Model file for the job. Use its own axes, mm. A direction names the side the tool comes from. Coordinates: 2 decimals unless noted, no trailing zeros. Loops run counter-clockwise (first coordinate to the right, second up) from the corner with the lowest first, then second, coordinate; pieces in that order, holes last.
from build123d import *
from build123d.topology import SkipClean

# Parameters (mm, degrees)
SKETCH1_R           = 6.35
BOSS_EXTRUDE1_DEPTH = 2.45
SKETCH2_R           = 1.5
BOSS_EXTRUDE2_DEPTH = 2.45
SKETCH3_R           = 2.85
CUT_EXTRUDE1_DEPTH  = 1.8
CHAMFER1_SIZE       = 5
CHAMFER1_SIZE2      = 3.501037691
BOSS_EXTRUDE3_DEPTH = 7.85


with BuildPart() as part:
    # Sketch1 → Boss-Extrude1 (new body)
    with BuildSketch(Plane(origin=(0, 0, 0), x_dir=(1, 0, 0), z_dir=(0, 1, 0))):
        with BuildLine():
            Line((-14.3, -17.6), (14.3, -17.6))
            Line((14.3, -17.6), (14.3, 5.715767665))
            ThreePointArc((14.3, 5.715767665), (0, 15.4), (-14.3, 5.715767665))
            Line((-14.3, 5.715767665), (-14.3, -17.6))
        make_face()
        with Locations(Location((0, 0, 0), (0, 0, 270))):
            Circle(SKETCH1_R, mode=Mode.SUBTRACT)
    extrude(amount=BOSS_EXTRUDE1_DEPTH)

    # Sketch2 → Boss-Extrude2 (add)
    with BuildSketch(Plane(origin=(0, 0, 0), x_dir=(1, 0, 0), z_dir=(0, 1, 0))):
        with BuildLine():
            ThreePointArc((24.104102849, -3.187555227), (26.549963246, 0.015574774), (24.073976981, 3.195475228))
            Line((24.073976981, 3.195475228), (14.3, 5.715767665))
            Line((14.3, 5.715767665), (14.3, -5.814556668))
            Line((14.3, -5.814556668), (24.104102849, -3.187555227))
        make_face()
        with Locations(Location((16.25, 0, 0), (0, 0, 270))):
            Circle(SKETCH2_R, mode=Mode.SUBTRACT)
        with Locations(Location((23.25, 0, 0), (0, 0, 270))):
            Circle(SKETCH2_R, mode=Mode.SUBTRACT)
    boss_extrude2 = extrude(amount=BOSS_EXTRUDE2_DEPTH)

    # Sketch3 → Cut-Extrude1 (cut)
    with BuildSketch(Plane(origin=(0, 2.45, 0), x_dir=(1, 0, 0), z_dir=(0, 1, 0))):
        with Locations(Location((16.25, 0, 0), (0, 0, 270))):
            Circle(SKETCH3_R)
    cut_extrude1 = extrude(amount=-CUT_EXTRUDE1_DEPTH, mode=Mode.SUBTRACT)

    # Mirror1: Boss-Extrude2, Cut-Extrude1 across plane
    add(boss_extrude2.mirror(Plane(origin=(0, 0, 0), x_dir=(0, 0, 1), z_dir=(1, 0, 0))))
    add(cut_extrude1.mirror(Plane(origin=(0, 0, 0), x_dir=(0, 0, 1), z_dir=(1, 0, 0))), mode=Mode.SUBTRACT)

    # Chamfer1
    chamfer1_edges = [part.edges().sort_by_distance(p)[0] for p in [
        (-14.3, 1.225, 17.6),
        (14.3, 1.225, 17.6),
    ]]
    chamfer1_side = [part.faces().sort_by_distance(p)[0] for p in [
        (0, 1.225, 17.6),
    ]]
    chamfer(chamfer1_edges, length=CHAMFER1_SIZE, length2=CHAMFER1_SIZE2, reference=chamfer1_side[0])

    # Sketch5 → Boss-Extrude3 (add)
    with BuildSketch(Plane(origin=(0, 2.45, 0), x_dir=(1, 0, 0), z_dir=(0, 1, 0))):
        with BuildLine():
            Line((14.3, 5.715767665), (14.3, -14.098962309))
            Line((14.3, -14.098962309), (9.3, -17.6))
            Line((9.3, -17.6), (6.7, -17.6))
            Line((6.7, -17.6), (6.7, -21.9))
            Line((6.7, -21.9), (0, -21.9))
            Line((0, -21.9), (0, -6.35))
            ThreePointArc((0, -6.35), (6.35, 0), (0, 6.35))
            Line((0, 6.35), (0, 15.4))
            ThreePointArc((0, 15.4), (8.63531059, 12.751133715), (14.3, 5.715767665))
        make_face()
    boss_extrude3 = extrude(amount=BOSS_EXTRUDE3_DEPTH)

    # Mirror2: Boss-Extrude3 across plane
    with SkipClean():  # the faces are left unmerged after this step: merging them gives an invalid solid
        add(boss_extrude3.mirror(Plane(origin=(0, 0, 0), x_dir=(0, 0, 1), z_dir=(1, 0, 0))))


solid = part.part
Q1. Slice it at B-B (x = 16.25). List the corners of the cut face in (y, z).
Answers:
outline: (0, -5.21) - (2.45, -5.21) - (2.45, -2.85) - (0.65, -2.85) - (0.65, -1.5) - (0, -1.5) - close; (0, 1.5) - (0.65, 1.5) - (0.65, 2.85) - (2.45, 2.85) - (2.45, 5.29) - (0, 5.29) - close
Q2. Slice it at D-D (z = 5). List the corners of the cut face in (x, y).
Answers:
outline: (-17.34, 0) - (-3.91, 0) - (-3.91, 10.3) - (-14.3, 10.3) - (-14.3, 2.45) - (-17.34, 2.45) - close; (3.91, 0) - (17.34, 0) - (17.34, 2.45) - (14.3, 2.45) - (14.3, 10.3) - (3.91, 10.3) - close
Q3. Mould opens along Z. For faces 5 (the flat face through (-19.255, 1.208, -4.438)), 6 (the flat face through (-11.84, 5.08, 15.82)), 7 (the cylindrical face through (17.515, 0.32, 0.806)) say: +Z half, -Z half, draft (parallel to the pull), parting line (faces both ways), or undercut.
Answers:
face 5: -Z half
face 6: +Z half
face 7: undercut
Q4. Flat gauge pins, fed straight in: P1, Ø3, axis at x = 17, z = 1, coming from the +Y side; P2, Ø16.5, axis at x = 0, z = 0, coming from the +Y side; P3, Ø9, axis at x = -22.5, z = -1.5, coming from the +Y side; P4, Ø4.5, axis at y = 7, z = 19, coming from the -X side. Where does each tip first touch, or does it go through?
Answers:
P1: stops at y = 0.65
P2: stops at y = 10.3
P3: stops at y = 2.45
P4: stops at x = -10.51
Q5. Which spindle directions (+Z, -Z, +X, -X, +Y, -Y) get a long thin tool onto all of the face, cutting with end or side? Do faces 1 (the flat face through (6.7, 6, 20)), 2 (the flat face through (0, 2.45, 20)), 3 (the cylindrical face through (-18.653, 1.563, 1.532)), 4 (the flat face through (-20, 2.45, 0)). Say none if no direction does.
Answers:
face 1: +Z, +X, +Y, -Y
face 2: +Z, +X, -X, -Y
face 3: none
face 4: +Z, -Z, -X, +Y
Q6. Drill centre lines: line 1 (X direction, y = 1.2, z = 0); line 2 (Z direction, x = 0, y = 3.25); line 3 (X direction, y = 1, z = 11). Where is each one in solid material? Low to high.
Answers:
line 1: x = -26.55 to -24.75, -21.75 to -19.1, -13.4 to -6.35, 6.35 to 13.4, 19.1 to 21.75, 24.75 to 26.55
line 2: z = -15.4 to -6.35, 6.35 to 21.9
line 3: x = -14.3 to 14.3
Q7. Slice it at C-C (y = 1.5). List the corners of the cut face in (x, z), and give its area (3 significant figures).
Answers:
outline: (-24.1, 3.19) arc R3.3 ccw to (-24.07, -3.2) - (-14.3, -5.72) arc R15.4 ccw to (14.3, -5.72) - (24.07, -3.2) arc R3.3 ccw to (24.1, 3.19) - (14.3, 5.81) - (14.3, 14.1) - (9.3, 17.6) - (-9.3, 17.6) - (-14.3, 14.1) - (-14.3, 5.81) - close; hole circle Ø3 at (-23.25, 0); hole circle Ø5.7 at (-16.25, 0); hole circle Ø12.7 at (0, 0); hole circle Ø5.7 at (16.25, 0); hole circle Ø3 at (23.25, 0)
area: 857 mm2
Q8. Slice it at A-A (y = 8.75). List the corners of the cut face in (x, z), and give its area (3 significant figures).
Answers:
outline: (-14.3, -5.72) arc R15.4 ccw to (14.3, -5.72) - (14.3, 14.1) - (9.3, 17.6) - (6.7, 17.6) - (6.7, 21.9) - (-6.7, 21.9) - (-6.7, 17.6) - (-9.3, 17.6) - (-14.3, 14.1) - close; hole circle Ø12.7 at (0, 0)
area: 781 mm2
